Autodesk Inventor part; units mm, degrees
ref_plane "YZ Plane" through (0, 0, 0) normal (1, 0, 0) x (0, 1, 0)
ref_plane "XZ Plane" through (0, 0, 0) normal (0, 1, 0) x (-1, 0, 0)
ref_plane "XY Plane" through (0, 0, 0) normal (0, 0, 1) x (1, 0, 0)
sketch "草图1" plane through (0, 0, 0) normal (0, 0, 1) x (1, 0, 0)
  line L0 (10, -4.6392) -> (-20.0603, -4.6392)
  line L1 (-20.0603, -4.6392) -> (-20.0603, 5.5)
  line L2 (-20.0603, 5.5) -> (10, 5.5)
  line L3 (10, 5.5) -> (10, -4.6392)
  point P0 (0, 0)
  dimension "d7" = 10.1392
extrude "拉伸1" add sketch "草图1" along normal blind 5.4
sketch "草图2" plane through (0, 0, 5.4) normal (0, 0, 1) x (1, 0, 0)
  circle A0 centre (5.3642, 2.7045) radius 1.5
  circle A1 centre (-15.4399, 2.7045) radius 1.5
extrude "拉伸2" cut sketch "草图2" against normal blind 21.65
properties part number "攻单夹片1"
Build history of the part. All positions in model axes, mm. Give positions to 0.01 mm unless a question says otherwise; leave off trailing zeros. Order: outer loops, then holes, each group sorted by start corner. A loop starts at its lowest first (then second) coordinate and runs counter-clockwise, first axis right, second up. Notation, with made-up numbers: M -9,-20 L 6,-20 A9 cw 6,-12 Z; hole C 56,-4.5 d3. An arc over 180 degrees is marked long. Use one line per item in the form item = value.
Q1. Slice it at C-C, the plane z = 2.3. Write the cut outline in (x, y).
Conclusion:
outline = M -20.06,-4.64 L 10,-4.64 L 10,5.5 L -20.06,5.5 Z; hole C -15.44,2.7 d3; hole C 5.36,2.7 d3
Q2. Slice it at B-B, the plane x = 6. Write the cut outline in (y, z).
Conclusion:
outline = M -4.64,0 L 1.35,0 L 1.35,5.4 L -4.64,5.4 Z; M 4.06,0 L 5.5,0 L 5.5,5.4 L 4.06,5.4 Z
Q3. Wall check: probe 1 along X at (y, z) = (1.75, 1.3); probe 2 along Y at (x, z) = (4, 3.05). Give the ranges that are in metal, low to high.
Conclusion:
probe_1 = -20.06 to -16.6, -14.28 to 4.21, 6.52 to 10
probe_2 = -4.64 to 2.08, 3.33 to 5.5
Q4. Pin check, flat tip, straight feed: P1, Ø1.8, axis at x = 5.36, y = 2.7, coming from the +Z side. Stop position of the tip, or through.
Conclusion:
P1 = through
Q5. Slice it at A-A, the plane y = 1.5. Write the cut outline in (x, z).
Conclusion:
outline = M -20.06,0 L -16.33,0 L -16.33,5.4 L -20.06,5.4 Z; M -14.55,0 L 4.47,0 L 4.47,5.4 L -14.55,5.4 Z; M 6.26,0 L 10,0 L 10,5.4 L 6.26,5.4 Z
Q6. Pull direction Y, two halves, no side cores. Call faces 1 (the flat face through (-5, 5.5, 3)), 2 (the cylindrical face through (-16.63, 1.79, 2.74)), 3 (the flat face through (-5, 1, 0)): released by +Y, released by -Y, zero draft, split by the parting line, or undercut.
Conclusion:
face_1 = released by +Y
face_2 = undercut
face_3 = zero draft
